Input: part model. Units: mm. Frame: model coordinates. A direction names the side the tool comes from. Round coordinates to 2 decimals unless told otherwise and drop trailing zeros. Loops run counter-clockwise (first coordinate to the right, second up) from the corner with the lowest first, then second, coordinate; pieces in that order, holes last.
1) Section B-B, the plane x = 5. State how many separate pieces and enclosed holes the cut face has, and give its area (3 significant figures).
2) Section C-C, the plane y = 5. Return loops of the section in (x, z).
3) Ray query, line 1 along X through (y, z) = (5, 9.75); line 2 along Y through (x, z) = (5, 89.2); line 3 along Y through (x, z) = (4, 8). Return the intervals inside material, ascending.
4) Section D-D, the plane z = 43.5. Return loops of the section in (x, y).
5) Draft query along X for faces 1 (the face through (12, -46, 46)), 2 (the face through (0, -34, 43)), 3 (the face through (5, 17, 5)). Return one class per face: pulls with the +X half, pulls with the -X half, needs draft (parallel to the pull), parting line crosses it, or undercut.
6) Section A-A, the plane y = 20. Return loops of the section in (x, z).
7) Access query for faces 4 (the face through (4.609, -70.735, 83.045)), 5 (the face through (4, 18, 3)), 6 (the face through (25, -34, 43)). Directions: +Z, -Z, +X, -X, +Y, -Y. A direction counts if a zero-diameter tool reaches every point of the face in a straight line with its end or side. Return the directions, or none.
8) First-contact query: pin 1 (5 mm diameter, centred on x = 5, y = 5, fed in from +Z); pin 2 (3 mm diameter, centred on x = 6, y = -74.5, fed in from -Z); pin 3 (5.5 mm diameter, centred on x = 6, y = -88, fed in from -Z). Flat tips, straight axial feed; report the tip coordinate or a pass-through.
from build123d import *

# Parameters (mm, degrees)
BOSS_EXTRUDE1_DEPTH = 25
CUT_EXTRUDE7_REACH  = 98.71
CUT_EXTRUDE7_START  = -3
SKETCH3_R           = 3
SKETCH3_R_2         = 1.6
CUT_EXTRUDE8_REACH  = 95.71
SKETCH3_3_R         = 1.6
CUT_EXTRUDE9_REACH  = 98.71
CUT_EXTRUDE9_START  = -3
SKETCH4_R           = 3
SKETCH4_R_2         = 1.6
CUT_EXTRUDE10_REACH = 95.71
SKETCH4_2_R         = 1.6


with BuildPart() as part:
    # Sketch1 → Boss-Extrude1 (new body)
    with BuildSketch(Plane(origin=(0, 0, 0), x_dir=(0, 0, -1), z_dir=(1, 0, 0))):
        Polygon((0, 0), (-93.70992099, -93.70992099), (-93.70992099, -68.70992099), (0, 25), align=None)
    extrude(amount=BOSS_EXTRUDE1_DEPTH)

    # Sketch3 → Cut-Extrude7 (cut, up to next)
    with BuildSketch(Plane(origin=(0, 0, 0), x_dir=(-1, 0, 0), z_dir=(0, 0, -1)).offset(CUT_EXTRUDE7_START), mode=Mode.PRIVATE) as cut_extrude7_sk1:
        with Locations((-20, 20)):
            Circle(SKETCH3_R)
        with Locations((-20, 20)):
            Circle(SKETCH3_R_2, mode=Mode.SUBTRACT)
    cut_extrude7_tool1 = extrude(cut_extrude7_sk1.sketch, amount=-CUT_EXTRUDE7_REACH, mode=Mode.PRIVATE) & part.part
    add(cut_extrude7_tool1.solids().sort_by_distance((22.915147, 20, 3))[0], mode=Mode.SUBTRACT)
    # Sketch3 → Cut-Extrude7 (cut, up to next)
    with BuildSketch(Plane(origin=(0, 0, 0), x_dir=(-1, 0, 0), z_dir=(0, 0, -1)).offset(CUT_EXTRUDE7_START), mode=Mode.PRIVATE) as cut_extrude7_sk2:
        with Locations((-20, 5)):
            Circle(SKETCH3_R)
        with Locations((-20, 5)):
            Circle(SKETCH3_R_2, mode=Mode.SUBTRACT)
    cut_extrude7_tool2 = extrude(cut_extrude7_sk2.sketch, amount=-CUT_EXTRUDE7_REACH, mode=Mode.PRIVATE) & part.part
    add(cut_extrude7_tool2.solids().sort_by_distance((22.915147, 5, 3))[0], mode=Mode.SUBTRACT)
    # Sketch3 → Cut-Extrude7 (cut, up to next)
    with BuildSketch(Plane(origin=(0, 0, 0), x_dir=(-1, 0, 0), z_dir=(0, 0, -1)).offset(CUT_EXTRUDE7_START), mode=Mode.PRIVATE) as cut_extrude7_sk3:
        with Locations((-5, 5)):
            Circle(SKETCH3_R)
        with Locations((-5, 5)):
            Circle(SKETCH3_R_2, mode=Mode.SUBTRACT)
    cut_extrude7_tool3 = extrude(cut_extrude7_sk3.sketch, amount=-CUT_EXTRUDE7_REACH, mode=Mode.PRIVATE) & part.part
    add(cut_extrude7_tool3.solids().sort_by_distance((7.915147, 5, 3))[0], mode=Mode.SUBTRACT)
    # Sketch3 → Cut-Extrude7 (cut, up to next)
    with BuildSketch(Plane(origin=(0, 0, 0), x_dir=(-1, 0, 0), z_dir=(0, 0, -1)).offset(CUT_EXTRUDE7_START), mode=Mode.PRIVATE) as cut_extrude7_sk4:
        with Locations((-5, 20)):
            Circle(SKETCH3_R)
        with Locations((-5, 20)):
            Circle(SKETCH3_R_2, mode=Mode.SUBTRACT)
    cut_extrude7_tool4 = extrude(cut_extrude7_sk4.sketch, amount=-CUT_EXTRUDE7_REACH, mode=Mode.PRIVATE) & part.part
    add(cut_extrude7_tool4.solids().sort_by_distance((7.915147, 20, 3))[0], mode=Mode.SUBTRACT)

    # Sketch3_3 → Cut-Extrude8 (cut, up to next)
    with BuildSketch(Plane(origin=(0, 0, 0), x_dir=(-1, 0, 0), z_dir=(0, 0, -1)), mode=Mode.PRIVATE) as cut_extrude8_sk1:
        with Locations((-20, 20)):
            Circle(SKETCH3_3_R)
    cut_extrude8_tool1 = extrude(cut_extrude8_sk1.sketch, amount=-CUT_EXTRUDE8_REACH, mode=Mode.PRIVATE) & part.part
    add(cut_extrude8_tool1.solids().sort_by_distance((20, 20, 0))[0], mode=Mode.SUBTRACT)
    # Sketch3_3 → Cut-Extrude8 (cut, up to next)
    with BuildSketch(Plane(origin=(0, 0, 0), x_dir=(-1, 0, 0), z_dir=(0, 0, -1)), mode=Mode.PRIVATE) as cut_extrude8_sk2:
        with Locations((-20, 5)):
            Circle(SKETCH3_3_R)
    cut_extrude8_tool2 = extrude(cut_extrude8_sk2.sketch, amount=-CUT_EXTRUDE8_REACH, mode=Mode.PRIVATE) & part.part
    add(cut_extrude8_tool2.solids().sort_by_distance((20, 5, 0))[0], mode=Mode.SUBTRACT)
    # Sketch3_3 → Cut-Extrude8 (cut, up to next)
    with BuildSketch(Plane(origin=(0, 0, 0), x_dir=(-1, 0, 0), z_dir=(0, 0, -1)), mode=Mode.PRIVATE) as cut_extrude8_sk3:
        with Locations((-5, 5)):
            Circle(SKETCH3_3_R)
    cut_extrude8_tool3 = extrude(cut_extrude8_sk3.sketch, amount=-CUT_EXTRUDE8_REACH, mode=Mode.PRIVATE) & part.part
    add(cut_extrude8_tool3.solids().sort_by_distance((5, 5, 0))[0], mode=Mode.SUBTRACT)
    # Sketch3_3 → Cut-Extrude8 (cut, up to next)
    with BuildSketch(Plane(origin=(0, 0, 0), x_dir=(-1, 0, 0), z_dir=(0, 0, -1)), mode=Mode.PRIVATE) as cut_extrude8_sk4:
        with Locations((-5, 20)):
            Circle(SKETCH3_3_R)
    cut_extrude8_tool4 = extrude(cut_extrude8_sk4.sketch, amount=-CUT_EXTRUDE8_REACH, mode=Mode.PRIVATE) & part.part
    add(cut_extrude8_tool4.solids().sort_by_distance((5, 20, 0))[0], mode=Mode.SUBTRACT)

    # Sketch4 → Cut-Extrude9 (cut, up to next)
    with BuildSketch(Plane.XY.offset(93.70992099).offset(CUT_EXTRUDE9_START), mode=Mode.PRIVATE) as cut_extrude9_sk1:
        with Locations((5, -73.70992099)):
            Circle(SKETCH4_R)
        with Locations((5, -73.70992099)):
            Circle(SKETCH4_R_2, mode=Mode.SUBTRACT)
    cut_extrude9_tool1 = extrude(cut_extrude9_sk1.sketch, amount=-CUT_EXTRUDE9_REACH, mode=Mode.PRIVATE) & part.part
    add(cut_extrude9_tool1.solids().sort_by_distance((2.084853, -73.709921, 90.709921))[0], mode=Mode.SUBTRACT)
    # Sketch4 → Cut-Extrude9 (cut, up to next)
    with BuildSketch(Plane.XY.offset(93.70992099).offset(CUT_EXTRUDE9_START), mode=Mode.PRIVATE) as cut_extrude9_sk2:
        with Locations((5, -88.70992099)):
            Circle(SKETCH4_R)
        with Locations((5, -88.70992099)):
            Circle(SKETCH4_R_2, mode=Mode.SUBTRACT)
    cut_extrude9_tool2 = extrude(cut_extrude9_sk2.sketch, amount=-CUT_EXTRUDE9_REACH, mode=Mode.PRIVATE) & part.part
    add(cut_extrude9_tool2.solids().sort_by_distance((2.084853, -88.709921, 90.709921))[0], mode=Mode.SUBTRACT)
    # Sketch4 → Cut-Extrude9 (cut, up to next)
    with BuildSketch(Plane.XY.offset(93.70992099).offset(CUT_EXTRUDE9_START), mode=Mode.PRIVATE) as cut_extrude9_sk3:
        with Locations((20, -88.70992099)):
            Circle(SKETCH4_R)
        with Locations((20, -88.70992099)):
            Circle(SKETCH4_R_2, mode=Mode.SUBTRACT)
    cut_extrude9_tool3 = extrude(cut_extrude9_sk3.sketch, amount=-CUT_EXTRUDE9_REACH, mode=Mode.PRIVATE) & part.part
    add(cut_extrude9_tool3.solids().sort_by_distance((17.084853, -88.709921, 90.709921))[0], mode=Mode.SUBTRACT)
    # Sketch4 → Cut-Extrude9 (cut, up to next)
    with BuildSketch(Plane.XY.offset(93.70992099).offset(CUT_EXTRUDE9_START), mode=Mode.PRIVATE) as cut_extrude9_sk4:
        with Locations((20, -73.70992099)):
            Circle(SKETCH4_R)
        with Locations((20, -73.70992099)):
            Circle(SKETCH4_R_2, mode=Mode.SUBTRACT)
    cut_extrude9_tool4 = extrude(cut_extrude9_sk4.sketch, amount=-CUT_EXTRUDE9_REACH, mode=Mode.PRIVATE) & part.part
    add(cut_extrude9_tool4.solids().sort_by_distance((17.084853, -73.709921, 90.709921))[0], mode=Mode.SUBTRACT)

    # Sketch4_2 → Cut-Extrude10 (cut, up to next)
    with BuildSketch(Plane.XY.offset(93.70992099), mode=Mode.PRIVATE) as cut_extrude10_sk1:
        with Locations((5, -73.70992099)):
            Circle(SKETCH4_2_R)
    cut_extrude10_tool1 = extrude(cut_extrude10_sk1.sketch, amount=-CUT_EXTRUDE10_REACH, mode=Mode.PRIVATE) & part.part
    add(cut_extrude10_tool1.solids().sort_by_distance((5, -73.709921, 93.709921))[0], mode=Mode.SUBTRACT)
    # Sketch4_2 → Cut-Extrude10 (cut, up to next)
    with BuildSketch(Plane.XY.offset(93.70992099), mode=Mode.PRIVATE) as cut_extrude10_sk2:
        with Locations((5, -88.70992099)):
            Circle(SKETCH4_2_R)
    cut_extrude10_tool2 = extrude(cut_extrude10_sk2.sketch, amount=-CUT_EXTRUDE10_REACH, mode=Mode.PRIVATE) & part.part
    add(cut_extrude10_tool2.solids().sort_by_distance((5, -88.709921, 93.709921))[0], mode=Mode.SUBTRACT)
    # Sketch4_2 → Cut-Extrude10 (cut, up to next)
    with BuildSketch(Plane.XY.offset(93.70992099), mode=Mode.PRIVATE) as cut_extrude10_sk3:
        with Locations((20, -88.70992099)):
            Circle(SKETCH4_2_R)
    cut_extrude10_tool3 = extrude(cut_extrude10_sk3.sketch, amount=-CUT_EXTRUDE10_REACH, mode=Mode.PRIVATE) & part.part
    add(cut_extrude10_tool3.solids().sort_by_distance((20, -88.709921, 93.709921))[0], mode=Mode.SUBTRACT)
    # Sketch4_2 → Cut-Extrude10 (cut, up to next)
    with BuildSketch(Plane.XY.offset(93.70992099), mode=Mode.PRIVATE) as cut_extrude10_sk4:
        with Locations((20, -73.70992099)):
            Circle(SKETCH4_2_R)
    cut_extrude10_tool4 = extrude(cut_extrude10_sk4.sketch, amount=-CUT_EXTRUDE10_REACH, mode=Mode.PRIVATE) & part.part
    add(cut_extrude10_tool4.solids().sort_by_distance((20, -73.709921, 93.709921))[0], mode=Mode.SUBTRACT)


solid = part.part
Final values:
1. separate pieces: 5
1. enclosed holes: 0
1. area: 2,080 mm2
2. outline: (0, 0) - (3.4, 0) - (3.4, 3) - (2, 3) - (2, 20) - (0, 20) - close; (6.6, 0) - (18.4, 0) - (18.4, 3) - (17, 3) - (17, 20) - (8, 20) - (8, 3) - (6.6, 3) - close; (21.6, 0) - (25, 0) - (25, 20) - (23, 20) - (23, 3) - (21.6, 3) - close
3. line 1: x = 0 to 2, 8 to 17, 23 to 25
3. line 2: y = -85.71 to -76.71, -70.71 to -64.2
3. line 3: y = -8 to 2.17, 7.83 to 17
4. outline: (0, -43.5) - (25, -43.5) - (25, -18.5) - (0, -18.5) - close
5. face 1: needs draft
5. face 2: pulls with the -X half
5. face 3: undercut
6. outline: (0, 0) - (3.4, 0) - (3.4, 3) - (2, 3) - (2, 5) - (0, 5) - close; (6.6, 0) - (18.4, 0) - (18.4, 3) - (17, 3) - (17, 5) - (8, 5) - (8, 3) - (6.6, 3) - close; (21.6, 0) - (25, 0) - (25, 5) - (23, 5) - (23, 3) - (21.6, 3) - close
7. face 4: -Z
7. face 5: +Z
7. face 6: +Z, -Z, +X, +Y, -Y
8. pin 1: stops at z = 3
8. pin 2: stops at z = 90.71
8. pin 3: stops at z = 85.25
